For this review, take the finished solid that the model builds, in its own axes (mm). Coordinates: 2 decimals unless noted, no trailing zeros.
1) We need section A-A on z = -407. Give the number of separate pieces and of enclosed holes in the cut face, then the cut area to 3 significant figures.
2) Insertion check: P1, Ø5.5, axis at y = -1, z = -135.5, coming from the +X side. The pin has a flat end and moves straight along its axis. Give the tip position at first contact, or say it passes through.
3) To check wall thickness, follow line 1 along X through (y, z) = (10.25, -82.5); line 2 along X through (y, z) = (2.5, -448). State the ranges of each line that lie inside material, in increasing order.
Autodesk Inventor part; units mm, degrees
ref_plane "YZ Plane" through (0, 0, 0) normal (1, 0, 0) x (0, 1, 0)
ref_plane "XZ Plane" through (0, 0, 0) normal (0, 1, 0) x (-1, 0, 0)
ref_plane "XY Plane" through (0, 0, 0) normal (0, 0, 1) x (1, 0, 0)
sketch "스케치1" plane through (0, 0, 0) normal (0, 0, 1) x (1, 0, 0)
  line L0 (-15, 15) -> (15, 15)
  line L1 (15, 15) -> (-15, 15)
  line L2 (-15, 15) -> (-15, -15)
  line L3 (-15, -15) -> (15, -15)
  line L4 (15, -15) -> (15, 15)
  line L5 (-15, -15) -> (-5, -15)
  line L6 (-5, -15) -> (-5, -5)
  line L7 (-5, -5) -> (-15, -5)
  line L8 (-15, -5) -> (-15, -15)
  line L9 (-15, 15) -> (-5, 15)
  line L10 (-5, 15) -> (-5, 5)
  line L11 (-5, 5) -> (-15, 5)
  line L12 (-15, 5) -> (-15, 15)
  line L13 (15, -15) -> (5, -15)
  line L14 (5, -15) -> (5, -5)
  line L15 (5, -5) -> (15, -5)
  line L16 (15, -5) -> (15, -15)
  line L17 (15, 15) -> (5, 15)
  line L18 (5, 15) -> (5, 5)
  line L19 (5, 5) -> (15, 5)
  line L20 (15, 5) -> (15, 15)
  line L21 (-13, -7) -> (-7, -7)
  line L22 (-7, -7) -> (-7, -13)
  line L23 (-7, -13) -> (-13, -13)
  line L24 (-13, -13) -> (-13, -7)
  line L25 (-13, 7) -> (-7, 7)
  line L26 (-7, 7) -> (-7, 13)
  line L27 (-7, 13) -> (-13, 13)
  line L28 (-13, 13) -> (-13, 7)
  line L29 (7, -7) -> (7, -13)
  line L30 (7, -13) -> (13, -13)
  line L31 (13, -13) -> (13, -7)
  line L32 (13, -7) -> (7, -7)
  line L33 (7, 7) -> (7, 13)
  line L34 (7, 13) -> (13, 13)
  line L35 (13, 13) -> (13, 7)
  line L36 (13, 7) -> (7, 7)
  line L37 (-5, -15) -> (-3, -15)
  line L38 (-3, -15) -> (-3, -13)
  line L39 (-3, -13) -> (-5, -13)
  line L40 (-5, -13) -> (-5, -15)
  line L41 (5, -15) -> (3, -15)
  line L42 (3, -15) -> (3, -13)
  line L43 (3, -13) -> (5, -13)
  line L44 (5, -13) -> (5, -15)
  line L45 (5, 15) -> (3, 15)
  line L46 (3, 15) -> (3, 13)
  line L47 (3, 13) -> (5, 13)
  line L48 (5, 13) -> (5, 15)
  line L49 (-5, 15) -> (-3, 15)
  line L50 (-3, 15) -> (-3, 13)
  line L51 (-3, 13) -> (-5, 13)
  line L52 (-5, 13) -> (-5, 15)
  line L53 (15, -5) -> (13, -5)
  line L54 (13, -5) -> (13, -3)
  line L55 (13, -3) -> (15, -3)
  line L56 (15, -3) -> (15, -5)
  line L57 (15, 5) -> (13, 5)
  line L58 (13, 5) -> (13, 3)
  line L59 (13, 3) -> (15, 3)
  line L60 (15, 3) -> (15, 5)
  line L61 (-15, -5) -> (-13, -5)
  line L62 (-13, -5) -> (-13, -3)
  line L63 (-13, -3) -> (-15, -3)
  line L64 (-15, -3) -> (-15, -5)
  line L65 (-15, 5) -> (-13, 5)
  line L66 (-13, 5) -> (-13, 3)
  line L67 (-13, 3) -> (-15, 3)
  line L68 (-15, 3) -> (-15, 5)
  line L69 (5, -5) -> (-5, -5)
  line L70 (-5, -5) -> (-5, 5)
  line L71 (-5, 5) -> (5, 5)
  line L72 (5, 5) -> (5, -5)
  line L73 (5, -5) -> (-5, 5) construction
  line L74 (-5, -5) -> (5, 5) construction
  line L75 (-3.5858, -5) -> (-5, -3.5858)
  line L76 (-5, -3.5858) -> (-6.4142, -5)
  line L77 (-6.4142, -5) -> (-5, -6.4142)
  line L78 (-5, -6.4142) -> (-3.5858, -5)
  line L79 (-3.5858, -5) -> (-6.4142, -5) construction
  line L80 (-5, -3.5858) -> (-5, -6.4142) construction
  line L81 (-3.5858, 5) -> (-5, 6.4142)
  line L82 (-5, 6.4142) -> (-6.4142, 5)
  line L83 (-6.4142, 5) -> (-5, 3.5858)
  line L84 (-5, 3.5858) -> (-3.5858, 5)
  line L85 (-3.5858, 5) -> (-6.4142, 5) construction
  line L86 (-5, 6.4142) -> (-5, 3.5858) construction
  line L87 (5, 3.5858) -> (6.4142, 5)
  line L88 (6.4142, 5) -> (5, 6.4142)
  line L89 (5, 6.4142) -> (3.5858, 5)
  line L90 (3.5858, 5) -> (5, 3.5858)
  line L91 (5, 3.5858) -> (5, 6.4142) construction
  line L92 (6.4142, 5) -> (3.5858, 5) construction
  line L93 (5, -3.5858) -> (6.4142, -5)
  line L94 (6.4142, -5) -> (5, -6.4142)
  line L95 (5, -6.4142) -> (3.5858, -5)
  line L96 (3.5858, -5) -> (5, -3.5858)
  line L97 (5, -3.5858) -> (5, -6.4142) construction
  line L98 (6.4142, -5) -> (3.5858, -5) construction
  line L99 (3, 3) -> (-3, 3)
  line L100 (-3, 3) -> (-3, -3)
  line L101 (-3, -3) -> (3, -3)
  line L102 (3, -3) -> (3, 3)
  point P0 (0, 0)
  point P1 (0, 0)
  point P2 (-10, 162)
  point P3 (-10, 162)
  point P4 (-10, 162)
  point P5 (-10, 162)
  point P6 (-18, 162)
  point P7 (-8, 152)
  point P8 (-10, 154)
  point P9 (0, 172)
  point P10 (0, 172)
  point P11 (0, 172)
  point P12 (0, 172)
  point P13 (8, 172)
  point P14 (10, 170)
  point P15 (-2, 182)
  point P16 (0, 180)
  point P17 (0, 162)
  point P18 (0, 162)
  point P19 (0, 162)
  point P20 (0, 162)
  point P21 (8, 162)
  point P22 (0, 154)
  point P23 (-2, 152)
  point P24 (10, 164)
  point P25 (-18, 172)
  point P26 (-10, 180)
  point P27 (-8, 182)
  point P28 (1.4142, 162)
  point P29 (0, 163.4142)
  point P30 (-1.4142, 162)
  point P31 (0, 160.5858)
  point P32 (0, 173.4142)
  point P33 (-1.4142, 172)
  point P34 (0, 170.5858)
  point P35 (1.4142, 172)
  point P36 (-11.4142, 172)
  point P37 (-10, 170.5858)
  point P38 (-8.5858, 172)
  point P39 (-10, 173.4142)
  point P40 (-10, 160.5858)
  point P41 (-8.5858, 162)
  point P42 (-10, 163.4142)
  point P43 (-11.4142, 162)
  point P44 (-18, 162)
  point P45 (-20, 162)
  point P46 (-10, 152)
  point P47 (-20, 182)
  point P48 (-20, 164)
  point P49 (-20, 164)
  point P50 (-20, 162)
  point P51 (-20, 170)
  point P52 (0, 0)
  point P53 (5, 15)
  dimension "d0" = 30
  dimension "d1" = 10
  dimension "d2" = 10
  dimension "d3" = 10
  dimension "d4" = 10
  dimension "d5" = 10
  dimension "d6" = 10
  dimension "d7" = 10
  dimension "d8" = 10
  dimension "d9" = 2
  dimension "d10" = 2
  dimension "d11" = 2
  dimension "d12" = 2
  dimension "d13" = 2
  dimension "d14" = 2
  dimension "d15" = 2
  dimension "d16" = 2
  dimension "d17" = 2
  dimension "d18" = 2
  dimension "d19" = 2
  dimension "d20" = 2
  dimension "d21" = 2
  dimension "d22" = 2
  dimension "d23" = 2
  dimension "d24" = 2
  dimension "d25" = 2
  dimension "d26" = 2
  dimension "d27" = 2
  dimension "d28" = 2
  dimension "d29" = 2
  dimension "d30" = 2
  dimension "d31" = 2
  dimension "d32" = 2
  dimension "d33" = 2
  dimension "d34" = 2
  dimension "d35" = 2
  dimension "d36" = 2
  dimension "d37" = 2
extrude "돌출1" add sketch "스케치1" against normal blind 540 contours L0 L10 L82 L11 L2 | L0 L50 L51 L10 | L11 L66 L67 L2 | L0 L18 L47 L46 | L81 L71 L10 | L10 L11 L82 | L63 L62 L7 L2 | L11 L70 L83 | L0 L4 L19 L88 L18 | L71 L84 L70 | L71 L90 L72 L96 L69 L75 L70 L84 | L7 L77 L6 L3 L2 | L89 L18 L71 | L71 L72 L90 | L75 L69 L70 | L70 L7 L76 | L4 L59 L58 L19 | L88 L19 L18 | L19 L87 L72 | L6 L39 L38 L3 | L7 L6 L77 | L69 L78 L6 | L93 L15 L72 | L72 L69 L96 | L69 L14 L95 | L4 L15 L54 L55 | L15 L94 L14 | L15 L4 L3 L14 L94 | L42 L43 L14 L3
properties part number "cross_AL_profile"
Result:
1. separate pieces: 1
1. enclosed holes: 5
1. area: 360 mm2
2. P1: stops at x = 15
3. line 1: x = -15 to -13, -7 to -5, 5 to 7, 13 to 15
3. line 2: x = -5 to -3, 3 to 5
